```python
from build123d import *

# Parameters (mm, degrees)
BOSS_EXTRUDE1_DEPTH = 5
CUT_EXTRUDE1_DEPTH  = 10


with BuildPart() as part:
    # Sketch1 → Boss-Extrude1 (new body)
    with BuildSketch(Plane.XY):
        Polygon((-84.25, 41.208366892), (-44.473549128, -49.25), (44.473549128, -49.25), (84.25, 41.208366892), (84.25, 49.25), (-84.25, 49.25), align=None)
    extrude(amount=BOSS_EXTRUDE1_DEPTH)

    # Sketch2 → Cut-Extrude1 (cut)
    with BuildSketch(Plane(origin=(0, 0, 0), x_dir=(-1, 0, 0), z_dir=(0, 0, -1))):
        Polygon((44.473549128, -49.25), (34.683249526, -34.25), (64.804143572, 34.25), (84.25, 41.208366892), align=None)
        Polygon((-64.804143572, 34.25), (-34.683249526, -34.25), (-44.473549128, -49.25), (-84.25, 41.208366892), align=None)
    extrude(amount=-CUT_EXTRUDE1_DEPTH, mode=Mode.SUBTRACT)


solid = part.part
```
Could you check a few things on this model? Use its own coordinates, in mm. A direction names the side the tool comes from. Round coordinates to 2 decimals unless told otherwise and drop trailing zeros. Write each loop counter-clockwise with the first axis right and the second up, starting at its lowest first coordinate (ties: lowest second). Pieces come first, ordered by that corner, then holes. Notation, with made-up numbers: M 14,58 L 35,58 A14 cw 35,62 Z; hole C -4,65 d9. An arc over 180 degrees is marked long. Answer in a Markdown table with one row per item. Add a question column.
Q1. Will this pin go through, and if not, where does the flat tip stop? pin 1 Ø3 at (y, z) = (-24, 1.5) entering from -X.
Q2. Imagine slicing it at C-C (y = 18). Please give me the cut outline in (x, z), then the cut area to 3 significant figures.
Q3. Imagine slicing it at D-D (x = 74.5). Please give me the cut outline in (y, z), then the cut area to 3 significant figures.
Q4. If we mould it in two halves opening along Y, with no side actions, what happens to faces 4 (the flat face through (84.25, 45, 2)), 5 (the flat face through (-1, -49.25, 2)), 6 (the flat face through (49.955, 0.48, 2.465))? For each: +Y half, -Y half, draft (parallel to the pull), parting line (faces both ways), or undercut.
Q5. Imagine slicing it at B-B (x = -36.5). Please give me the cut outline in (y, z), then the cut area to 3 significant figures.
Q6. Imagine slicing it at A-A (z = 1.25). Please give me the cut outline in (x, y), then the cut area to 3 significant figures.
Q7. If I drill on line 1 (Y direction, x = 38, z = 3.85); line 2 (X direction, y = 32, z = 1.5); line 3 (X direction, y = 20.5, z = 3.1), over which ranges is the centre line in solid material (lowest first)? Write a range as from..to.
Q8. On a 3-axis mill with a long thin cutter (end or side, diameter ignored), from which of +Z, -Z, +X, -X, +Y, -Y can I reach the whole of each face in a straight line? I mean faces 1 (the flat face through (-1, 12, 5)), 2 (the flat face through (-49.533, -0.48, 2.465)), 3 (the flat face through (39.51, -41.645, 2.465)). Say none if no direction works.
Values:
| question | item | result |
|---|---|---|
| 1 | pin 1 | x = -39.85 |
| 2 | outline | M -57.66,0 L 57.66,0 L 57.66,5 L -57.66,5 Z |
| 2 | area | 577 mm^2 |
| 3 | outline | M 37.72,0 L 49.25,0 L 49.25,5 L 37.72,5 Z |
| 3 | area | 57.7 mm^2 |
| 4 | face 4 | draft |
| 4 | face 5 | -Y half |
| 4 | face 6 | undercut |
| 5 | outline | M -49.25,0 L -37.03,0 L -37.03,5 L -49.25,5 Z; M -30.12,0 L 49.25,0 L 49.25,5 L -30.12,5 Z |
| 5 | area | 458 mm^2 |
| 6 | outline | M -84.25,41.21 L -64.8,34.25 L -34.68,-34.25 L -44.47,-49.25 L 44.47,-49.25 L 34.68,-34.25 L 64.8,34.25 L 84.25,41.21 L 84.25,49.25 L -84.25,49.25 Z |
| 6 | area | 10,400 mm^2 |
| 7 | line 1 | -49.25..-39.33, -26.71..49.25 |
| 7 | line 2 | -63.81..63.81 |
| 7 | line 3 | -58.76..58.76 |
| 8 | face 1 | +Z, +X, -X, +Y, -Y |
| 8 | face 2 | +Z, -Z, -X |
| 8 | face 3 | +Z, -Z, +X |
